Work out the finished part from the listing and answer in its coordinate system (mm). Coordinates: 2 decimals unless noted, no trailing zeros. Order: outer loops, then holes, each group sorted by start corner. A loop starts at its lowest first (then second) coordinate and runs counter-clockwise, first axis right, second up.
1. Flat-ended cylindrical pins translate along their axes: pin 1 Ø2 at (x, z) = (27, 1) entering from -Y; pin 2 Ø3 at (x, z) = (0, 3) entering from -Y; pin 3 Ø1.8 at (y, z) = (-17, 2.5) entering from +X. Find the tip coordinate at first contact, or state that the pin passes through.
2. The part is cut by section D-D, the plane z = 3.1. Count the separate pieces of the cut face and the enclosed holes in it, then the cut area to 3 significant figures.
3. Find the intervals of material crossed by probe 1 along Y at (x, z) = (-29, 3.95); probe 2 along X at (y, z) = (14.5, 3.6); probe 3 along X at (y, z) = (-9, 4.05), in increasing order.
4. The part is cut by section A-A, the plane x = 0. Give the vertices of the cut face in (y, z), then the cut area to 3 significant figures.
5. The part is cut by section B-B, the plane y = -3.5. Give the vertices of the cut face in (x, z), then the cut area to 3 significant figures.
6. The part is cut by section C-C, the plane x = 10.5. Give the vertices of the cut face in (y, z).
7. Determine the mould class of faces 1 (the flat face through (-19.15, 16, 3)), 2 (the cylindrical face through (-37.664, 11.861, 2.88)), 3 (the flat face through (-1, -17, 5.842)) for opening direction Y: +Y half, -Y half, draft (parallel to the pull), parting line (faces both ways), or undercut.
```python
from build123d import *

# Parameters (mm, degrees)
SKETCH1_R           = 41.275
SKETCH1_R_2         = 3.175
BOSS_EXTRUDE1_DEPTH = 5.842
SKETCH7_R           = 41.275
SKETCH7_R_2         = 39.487499946
CUT_EXTRUDE3_DEPTH  = 59.663278241
SKETCH8_W           = 5.842
SKETCH8_H           = 12.7
SKETCH8_W_2         = 12.7
SKETCH8_H_2         = 5.842
CUT_EXTRUDE4_DEPTH  = 57.148501921


with BuildPart() as part:
    # Sketch1 → Boss-Extrude1 (new body)
    with BuildSketch(Plane.XY):
        Circle(SKETCH1_R)
        with Locations((0, 34.925)):
            Circle(SKETCH1_R_2, mode=Mode.SUBTRACT)
        with Locations((30.245937227, -17.4625)):
            Circle(SKETCH1_R_2, mode=Mode.SUBTRACT)
        with Locations((-30.245937227, -17.4625)):
            Circle(SKETCH1_R_2, mode=Mode.SUBTRACT)
        with BuildLine():
            Line((-25.3015625, -12.8), (25.3015625, -12.8))
            ThreePointArc((25.3015625, -12.8), (25.640316502, -12.940316502), (25.5, -12.6015625))
            Line((25.5, -12.6015625), (25.5, 12.6015625))
            ThreePointArc((25.5, 12.6015625), (25.640316502, 12.940316502), (25.3015625, 12.8))
            Line((25.3015625, 12.8), (-25.3015625, 12.8))
            ThreePointArc((-25.3015625, 12.8), (-25.640316502, 12.940316502), (-25.5, 12.6015625))
            Line((-25.5, 12.6015625), (-25.5, -12.6015625))
            ThreePointArc((-25.5, -12.6015625), (-25.640316502, -12.940316502), (-25.3015625, -12.8))
        make_face(mode=Mode.SUBTRACT)
    extrude(amount=BOSS_EXTRUDE1_DEPTH)

    # Sketch7 → Cut-Extrude3 (cut, through all)
    with BuildSketch(Plane(origin=(0, 0, 0), x_dir=(-1, 0, 0), z_dir=(0, 0, -1))):
        Circle(SKETCH7_R)
        Circle(SKETCH7_R_2, mode=Mode.SUBTRACT)
    extrude(amount=-CUT_EXTRUDE3_DEPTH, mode=Mode.SUBTRACT)

    # Sketch8 → Cut-Extrude4 (cut, through all)
    with BuildSketch(Plane(origin=(0, 0, 0), x_dir=(-1, 0, 0), z_dir=(0, 0, -1))):
        with Locations((-28.421, 0)):
            Rectangle(SKETCH8_W, SKETCH8_H)
        with Locations((-12.599996942, 15.721)):
            Rectangle(SKETCH8_W_2, SKETCH8_H_2)
        with Locations((12.800003058, 15.721)):
            Rectangle(SKETCH8_W_2, SKETCH8_H_2)
        with Locations((12.800003058, -15.721)):
            Rectangle(SKETCH8_W_2, SKETCH8_H_2)
        with Locations((-12.599996942, -15.721)):
            Rectangle(SKETCH8_W_2, SKETCH8_H_2)
        with Locations((28.421, 0)):
            Rectangle(SKETCH8_W, SKETCH8_H)
    extrude(amount=-CUT_EXTRUDE4_DEPTH, mode=Mode.SUBTRACT)


solid = part.part
```
Geometry says:
1. pin 1: stops at y = -29.72
1. pin 2: stops at y = -39.49
1. pin 3: stops at x = 36.06
2. separate pieces: 1
2. enclosed holes: 4
2. area: 3,050 mm2
3. probe 1: y = -26.8 to -20.38, -14.54 to -6.35, 6.35 to 26.8
3. probe 2: x = -36.73 to -19.15, -6.45 to 6.25, 18.95 to 36.73
3. probe 3: x = -38.45 to -25.5, 25.5 to 38.45
4. outline: (-39.49, 0) - (-12.8, 0) - (-12.8, 5.84) - (-39.49, 5.84) - close; (12.8, 0) - (31.75, 0) - (31.75, 5.84) - (12.8, 5.84) - close; (38.1, 0) - (39.49, 0) - (39.49, 5.84) - (38.1, 5.84) - close
4. area: 275 mm2
5. outline: (-39.33, 0) - (-31.34, 0) - (-31.34, 5.84) - (-39.33, 5.84) - close; (31.34, 0) - (39.33, 0) - (39.33, 5.84) - (31.34, 5.84) - close
5. area: 93.4 mm2
6. outline: (-38.07, 0) - (-18.64, 0) - (-18.64, 5.84) - (-38.07, 5.84) - close; (18.64, 0) - (38.07, 0) - (38.07, 5.84) - (18.64, 5.84) - close
7. face 1: undercut
7. face 2: parting line
7. face 3: draft
